from build123d import *

# Parameters (mm, degrees)
BOSS_EXTRUDE1_DEPTH = 16
SKETCH2_4_W         = 74
SKETCH2_4_H         = 76
BOSS_EXTRUDE2_DEPTH = 2
SKETCH3_W           = 2
SKETCH3_H           = 4
SKETCH3_H_2         = 8
BOSS_EXTRUDE3_DEPTH = 76
LPATTERN1_COUNT     = 2
LPATTERN1_PITCH     = 72
SKETCH4_W           = 2
SKETCH4_H           = 4
SKETCH4_H_2         = 8
BOSS_EXTRUDE5_DEPTH = 71
FILLET2_R           = 5
SKETCH7_R           = 2
BOSS_EXTRUDE9_DEPTH = 3.5
SKETCH8_W           = 60
SKETCH8_H           = 1
CUT_EXTRUDE1_DEPTH  = 2
FILLET12_R          = 1
SKETCH11_W          = 2
SKETCH11_H          = 1.5
CUT_EXTRUDE2_DEPTH  = 112.462998345
SKETCH12_W          = 2
SKETCH12_H          = 1.5
CUT_EXTRUDE3_DEPTH  = 111.072703247
FILLET13_R          = 8
FILLET14_R          = 1
FILLET16_R          = 0.5


# Some blends are built 0.0001 mm under size
with BuildPart() as part:
    # Sketch2 → Boss-Extrude1 (new body)
    with BuildSketch(Plane(origin=(0, 0, 0), x_dir=(1, 0, 0), z_dir=(0, 1, 0))):
        Polygon((-78, 0), (-76, 0), (-76, 76), (-2, 76), (-2, 0), (0, 0), (0, 78), (-78, 78), align=None)
    extrude(amount=BOSS_EXTRUDE1_DEPTH)

    # Sketch2<4> → Boss-Extrude2 (add)
    with BuildSketch(Plane(origin=(0, 0, 0), x_dir=(1, 0, 0), z_dir=(0, 1, 0))):
        with Locations((-39, 38)):
            Rectangle(SKETCH2_4_W, SKETCH2_4_H)
    extrude(amount=BOSS_EXTRUDE2_DEPTH)

    # Sketch3 → Boss-Extrude3 (add)
    with BuildSketch(Plane.XY):
        with Locations((-75, 14)):
            Rectangle(SKETCH3_W, SKETCH3_H)
        with Locations((-75, 6)):
            Rectangle(SKETCH3_W, SKETCH3_H_2)
    boss_extrude3 = extrude(amount=-BOSS_EXTRUDE3_DEPTH)

    # LPattern1: Boss-Extrude3 ×2
    with Locations(*[(i * LPATTERN1_PITCH, 0, 0) for i in range(1, LPATTERN1_COUNT)]):
        add(boss_extrude3)

    # Sketch4 → Boss-Extrude5 (add)
    with BuildSketch(Plane(origin=(-74, 0, 0), x_dir=(0, 0, -1), z_dir=(1, 0, 0))):
        with Locations((75, 14)):
            Rectangle(SKETCH4_W, SKETCH4_H)
        with Locations((75, 6)):
            Rectangle(SKETCH4_W, SKETCH4_H_2)
    extrude(amount=BOSS_EXTRUDE5_DEPTH)

    # Fillet2
    fillet2_edges = [part.edges().sort_by_distance(p)[0] for p in [
        (-74, 14, -74),
        (-4, 6, -74),
        (-74, 6, -74),
        (-76, 11, -76),
        (-2, 11, -76),
        (-4, 14, -74),
    ]]
    fillet(fillet2_edges, radius=FILLET2_R)

    # Sketch7 → Boss-Extrude9 (add)
    # profile 1 of 4: a face of its own
    with BuildSketch(Plane(origin=(0, 2, 0), x_dir=(1, 0, 0), z_dir=(0, 1, 0))):
        with BuildLine():
            Line((-66.5, 74.491060011), (-74, 74.491060011))
            Line((-74, 74.491060011), (-74, 67.5))
            Line((-74, 67.5), (-70, 67.5))
            ThreePointArc((-70, 67.5), (-67.525126266, 68.525126266), (-66.5, 71))
            Line((-66.5, 71), (-66.5, 74.491060011))
        make_face()
        with Locations(Location((-70, 71, 0), (0, 0, 270))):
            Circle(SKETCH7_R, mode=Mode.SUBTRACT)
    # profile 2 of 4: a face of its own
    with BuildSketch(Plane(origin=(0, 2, 0), x_dir=(1, 0, 0), z_dir=(0, 1, 0))):
        with BuildLine():
            ThreePointArc((-11.5, 71), (-10.474873734, 68.525126266), (-8, 67.5))
            Line((-8, 67.5), (-4, 67.5))
            Line((-4, 67.5), (-4, 74.5))
            Line((-4, 74.5), (-11.5, 74.5))
            Line((-11.5, 74.5), (-11.5, 71))
        make_face()
        with Locations(Location((-8, 71, 0), (0, 0, 270))):
            Circle(SKETCH7_R, mode=Mode.SUBTRACT)
    # profile 3 of 4: a face of its own
    with BuildSketch(Plane(origin=(0, 2, 0), x_dir=(1, 0, 0), z_dir=(0, 1, 0))):
        with BuildLine():
            Line((-74, 5.5), (-70, 5.5))
            ThreePointArc((-70, 5.5), (-66.5, 9), (-70, 12.5))
            Line((-70, 12.5), (-74, 12.5))
            Line((-74, 12.5), (-74, 5.5))
        make_face()
        with Locations(Location((-70, 9, 0), (0, 0, 270))):
            Circle(SKETCH7_R, mode=Mode.SUBTRACT)
    # profile 4 of 4: a face of its own
    with BuildSketch(Plane(origin=(0, 2, 0), x_dir=(1, 0, 0), z_dir=(0, 1, 0))):
        with BuildLine():
            Line((-4, 12.5), (-8, 12.5))
            ThreePointArc((-8, 12.5), (-11.5, 9), (-8, 5.5))
            Line((-8, 5.5), (-4, 5.5))
            Line((-4, 5.5), (-4, 12.5))
        make_face()
        with Locations(Location((-8, 9, 0), (0, 0, 270))):
            Circle(SKETCH7_R, mode=Mode.SUBTRACT)
    extrude(amount=BOSS_EXTRUDE9_DEPTH)

    # Sketch8 → Cut-Extrude1 (cut)
    with BuildSketch(Plane.XY.offset(-74)):
        with Locations((-39, 9.5)):
            Rectangle(SKETCH8_W, SKETCH8_H)
    extrude(amount=-CUT_EXTRUDE1_DEPTH, mode=Mode.SUBTRACT)

    # Fillet12
    fillet12_edges = [part.edges().sort_by_distance(p)[0] for p in [
        (-9, 9, -75),
        (-69, 9, -75),
        (-39, 9, -76),
    ]]
    fillet(fillet12_edges, radius=FILLET12_R - 0.0001)  # a hair under: the kernel refuses the full size

    # Sketch11 → Cut-Extrude2 (cut, through all)
    with BuildSketch(Plane.XY):
        with Locations((-77, 15.25)):
            Rectangle(SKETCH11_W, SKETCH11_H)
        with Locations((-1, 15.25)):
            Rectangle(SKETCH11_W, SKETCH11_H)
    extrude(amount=-CUT_EXTRUDE2_DEPTH, mode=Mode.SUBTRACT)

    # Sketch12 → Cut-Extrude3 (cut, through all)
    with BuildSketch(Plane.ZY.offset(76)):
        with Locations((-77, 15.25)):
            Rectangle(SKETCH12_W, SKETCH12_H)
    extrude(amount=-CUT_EXTRUDE3_DEPTH, mode=Mode.SUBTRACT)

    # Fillet13
    # the kernel refuses this fillet: 8 mm, written as the material it takes off along each edge
    with BuildSketch(Plane(origin=(-78, -20, -78), x_dir=(0, 0, 1), z_dir=(0, 1, 0)), Plane(origin=(0, -20, -78), x_dir=(-1, 0, 0), z_dir=(0, 1, 0)), Plane(origin=(-78, -20, 0), x_dir=(1, 0, 0), z_dir=(0, 1, 0))) as fillet13_piece_1:
        with BuildLine():
            CenterArc((FILLET13_R, FILLET13_R), FILLET13_R, 180, 90)
            Line((0, FILLET13_R), (0, 0))
            Line((0, 0), (FILLET13_R, 0))
        make_face()
    extrude(amount=54.5, mode=Mode.SUBTRACT)
    with BuildSketch(Plane(origin=(-76, 36, -76), x_dir=(0, 0, 1), z_dir=(0, -1, 0)), Plane(origin=(-2, 36, -76), x_dir=(-1, 0, 0), z_dir=(0, -1, 0))) as fillet13_piece_2:
        with BuildLine():
            CenterArc((FILLET13_R, -FILLET13_R), FILLET13_R, 90, 90)
            Line((0, -FILLET13_R), (0, 0))
            Line((0, 0), (FILLET13_R, 0))
        make_face()
    extrude(amount=21.5, mode=Mode.SUBTRACT)
    with BuildSketch(Plane(origin=(0, -20, 0), x_dir=(-1, 0, 0), z_dir=(0, 1, 0))) as fillet13_piece_3:
        with BuildLine():
            CenterArc((FILLET13_R, -FILLET13_R), FILLET13_R, 90, 90)
            Line((0, -FILLET13_R), (0, 0))
            Line((0, 0), (FILLET13_R, 0))
        make_face()
    extrude(amount=54.5, mode=Mode.SUBTRACT)

    # Fillet14
    fillet14_edges = [part.edges().sort_by_distance(p)[0] for p in [
        (-39, 16, -76),
        (-76, 16, -35.354248689),
        (-2, 16, -35.354248689),
        (-4.343145751, 16, -73.656854249),
        (-73.656854249, 16, -73.656854249),
    ]]
    fillet(fillet14_edges, radius=FILLET14_R)

    # Fillet16
    # the kernel refuses this fillet: 0.5 mm, written as the material it takes off along each edge
    with BuildSketch(Plane(origin=(-74, 10, 0.17820323), x_dir=(0, -1, 0), z_dir=(0, 0, -1)), Plane(origin=(-4, 10, 0.17820323), x_dir=(1, 0, 0), z_dir=(0, 0, -1)), Plane(origin=(-4, 12, 0.17820323), x_dir=(0, 1, 0), z_dir=(0, 0, -1)), Plane(origin=(-74, 12, 0.17820323), x_dir=(-1, 0, 0), z_dir=(0, 0, -1))) as fillet16_piece_1:
        with BuildLine():
            CenterArc((FILLET16_R, FILLET16_R), FILLET16_R, 180, 90)
            Line((0, FILLET16_R), (0, 0))
            Line((0, 0), (FILLET16_R, 0))
        make_face()
    extrude(amount=69.17820323, mode=Mode.SUBTRACT)
    with BuildSketch(Plane(origin=(-69, 12, -74), x_dir=(0, 0, -1), z_dir=(1, 0, 0))) as fillet16_piece_2:
        with BuildLine():
            CenterArc((FILLET16_R, FILLET16_R), FILLET16_R, 180, 90)
            Line((0, FILLET16_R), (0, 0))
            Line((0, 0), (FILLET16_R, 0))
        make_face()
    extrude(amount=60, mode=Mode.SUBTRACT)
    with BuildSketch(Plane(origin=(-9, 12, -69), x_dir=(1, 0, 0), z_dir=(0, 0, 1))) as fillet16_piece_3:
        with BuildLine():
            CenterArc((5 + FILLET16_R, FILLET16_R), FILLET16_R, 180, 90)
            Line((5, FILLET16_R), (5, 0))
            Line((5, 0), (5 + FILLET16_R, 0))
        make_face()
    revolve(axis=Axis((-9, 12, -69), (0, 1, 0)), revolution_arc=90, mode=Mode.SUBTRACT)
    with BuildSketch(Plane(origin=(-9, 10, -69), x_dir=(1, 0, 0), z_dir=(0, 0, 1))) as fillet16_piece_4:
        with BuildLine():
            CenterArc((5 + FILLET16_R, -FILLET16_R), FILLET16_R, 90, 90)
            Line((5, -FILLET16_R), (5, 0))
            Line((5, 0), (5 + FILLET16_R, 0))
        make_face()
    revolve(axis=Axis((-9, 10, -69), (0, 1, 0)), revolution_arc=104.329698924, mode=Mode.SUBTRACT)
    with BuildSketch(Plane(origin=(-69, 12, -69), x_dir=(0, 0, -1), z_dir=(1, 0, 0))) as fillet16_piece_5:
        with BuildLine():
            CenterArc((5 + FILLET16_R, FILLET16_R), FILLET16_R, 180, 90)
            Line((5, FILLET16_R), (5, 0))
            Line((5, 0), (5 + FILLET16_R, 0))
        make_face()
    revolve(axis=Axis((-69, 12, -69), (0, 1, 0)), revolution_arc=90, mode=Mode.SUBTRACT)
    with BuildSketch(Plane(origin=(-69, 10, -69), x_dir=(0.24750126301206582, 0, -0.9688875707776585), z_dir=(0.9688875707776585, 0, 0.24750126301206582))) as fillet16_piece_6:
        with BuildLine():
            CenterArc((5 + FILLET16_R, -FILLET16_R), FILLET16_R, 90, 90)
            Line((5, -FILLET16_R), (5, 0))
            Line((5, 0), (5 + FILLET16_R, 0))
        make_face()
    revolve(axis=Axis((-69, 10, -69), (0, 1, 0)), revolution_arc=104.329698924, mode=Mode.SUBTRACT)


solid = part.part
Build history of the part. All positions in model axes, mm. A direction names the side the tool comes from. Coordinates: 2 decimals unless noted, no trailing zeros. Order: outer loops, then holes, each group sorted by start corner. A loop starts at its lowest first (then second) coordinate and runs counter-clockwise, first axis right, second up. Notation, with made-up numbers: M -36.5,-6 L 21.5,-6 A18 ccw 21.5,1 Z; hole C -16.5,84.5 d7. An arc over 180 degrees is marked long. One line per question, with ' | ' between items. Start each with the question number.
Q1. Saw through at B-B (y = 4). List the corners of the cut face in (x, z).
Q2. Saw through at A-A (x = -41.5). List the corners of the cut face in (y, z), then the cut area to 3 significant figures.
Q3. 3-axis set-ups, long thin cutter, end or side, ignore diameter. For faces 3 (the face through (-39.2, 14.5, -76.4)), 4 (the face through (-8, 2, -71)), 5 (the face through (-11.5, 4, -73)), 6 (the face through (-75, 12, -41)): which of +Z, -Z, +X, -X, +Y, -Y reach the whole face in a straight line?
Q4. Flat gauge pins, fed straight in: pin 1 Ø5 at (x, y) = (-36, 9) entering from +Z; pin 2 Ø8 at (x, y) = (-8.5, 9) entering from +Z; pin 3 Ø2.5 at (y, z) = (4, -72.5) entering from +X. Where does each tip first touch, or does it go through?
Q5. Two-plate mould, pull along X, no slides. Class faces 1 (the face through (-39, 5, -74)), 2 (the face through (-39, 7, -78)): +X half, -X half, draft (parallel to the pull), parting line (faces both ways), or undercut.
Q6. Saw through at C-C (z = -40). List the corners of the cut face in (x, y), then the cut area to 3 significant figures.
Q7. Probe L1, parallel to X at y = 3.3, z = -9; L2, parallel to X at y = 12.75, z = -33.5; L3, parallel to X at y = 10.25, z = -51.5. List the from-to ranges inside material, lowest first. Write a range as from..to.
Check values:
1) outline: M -78,-70 A8 ccw -70,-78 L -8,-78 A8 ccw 0,-70 L 0,-8 A8 ccw -4,-1.07 L -4,-5.5 L -8,-5.5 A3.5 ccw -8,-12.5 L -4,-12.5 L -4,-67.5 L -8,-67.5 A3.5 ccw -11.5,-71 L -11.5,-74 L -66.5,-74 L -66.5,-71 A3.5 ccw -70,-67.5 L -74,-67.5 L -74,-12.5 L -70,-12.5 A3.5 ccw -70,-5.5 L -74,-5.5 L -74,-1.07 A8 ccw -78,-8 Z; hole C -70,-71 d4; hole C -70,-9 d4; hole C -8,-71 d4; hole C -8,-9 d4
2) outline: M 0,-78 L 14.5,-78 L 14.5,-76 L 15,-76 A1 ccw 16,-75 L 16,-74 L 12.5,-74 A0.5 ccw 12,-74.5 L 12,-76 L 10,-76 A1 cw 9,-75 L 9,-74 L 2,-74 L 2,0 L 0,0 Z | area: 203 mm2
3) face 3: -Z, +Y | face 4: +Y | face 5: +Z, +Y | face 6: +Z
4) pin 1: stops at z = -74 | pin 2: stops at z = -5.5 | pin 3: stops at x = -0.1
5) face 1: undercut | face 2: draft
6) outline: M -78,0 L 0,0 L 0,14.5 L -2,14.5 L -2,15 A1 ccw -3,16 L -4,16 L -4,12.5 A0.5 ccw -3.5,12 L -2,12 L -2,10 L -3.5,10 A0.5 ccw -4,9.5 L -4,2 L -74,2 L -74,9.5 A0.5 ccw -74.5,10 L -76,10 L -76,12 L -74.5,12 A0.5 ccw -74,12.5 L -74,16 L -75,16 A1 ccw -76,15 L -76,14.5 L -78,14.5 Z | area: 253 mm2
7) L1: x = -78..-72, -68..-66.5, -11.5..-10, -6..0 | L2: x = -78..-74, -4..0 | L3: x = -78..-76, -2..0
